```python
from build123d import *

# Parameters (mm, degrees)
SKETCH_W        = 90
SKETCH_H        = 130
PAD_DEPTH       = 3
PAD007_DEPTH    = 3
PAD006_DEPTH    = 3
SKETCH009_W     = 90
SKETCH009_H     = 130
PAD008_DEPTH    = 2
SKETCH010_R     = 19.0420352847
POCKET_DEPTH    = 10
CHAMFER_SIZE    = 1
SKETCH011_W     = 90
SKETCH011_H     = 4
POCKET001_DEPTH = 5


with BuildPart() as pad007:
    # Sketch → Pad (new body)
    with BuildSketch(Plane.XY):
        with Locations((45, 65)):
            Rectangle(SKETCH_W, SKETCH_H)
    extrude(amount=PAD_DEPTH)

    # Sketch006 → Pad007 (new body)
    with BuildSketch(Plane.XY.offset(3)):
        with BuildLine():
            Line((0, 0), (90, 0))
            Line((90, 0), (90, 31.200001))
            Line((90, 87.7297593266), (90, 31.200001))
            Line((63.384261619, 87.7297593266), (90, 87.7297593266))
            ThreePointArc((73.2419105019, 65.6401585516), (70.414665309, 77.6228043326), (63.384261619, 87.7297593266))
            ThreePointArc((61.470024, 41.9983394519), (70.1525128312, 52.4267750542), (73.2419105019, 65.6401585516))
            Line((61.470024, 31.2), (61.470024, 41.9983394519))
            Line((0, 31.2), (61.470024, 31.2))
            Line((0, 31.2), (0, 0))
        make_face()
    extrude(amount=PAD007_DEPTH)


with BuildPart() as pocket001:
    # Sketch008 → Pad006 (new body)
    with BuildSketch(Plane(origin=(90, 130, 3), x_dir=(-1, 0, 0), z_dir=(0, 0, 1))):
        with BuildLine():
            Line((0, 0), (90, 0))
            Line((90, 0), (90, 31.200001))
            Line((90, 87.7297593266), (90, 31.200001))
            Line((63.384261619, 87.7297593266), (90, 87.7297593266))
            ThreePointArc((73.2419105019, 65.6401585516), (70.414665309, 77.6228043326), (63.384261619, 87.7297593266))
            ThreePointArc((61.470024, 41.9983394519), (70.1525128312, 52.4267750542), (73.2419105019, 65.6401585516))
            Line((61.470024, 31.2), (61.470024, 41.9983394519))
            Line((0, 31.2), (61.470024, 31.2))
            Line((0, 31.2), (0, 0))
        make_face()
    extrude(amount=PAD006_DEPTH)

    # Fusion: union Pad007
    add(pad007.part)

    # Sketch009 → Pad008 (new body)
    with BuildSketch(Plane.XY.offset(6)):
        with Locations((45, 65)):
            Rectangle(SKETCH009_W, SKETCH009_H)
    extrude(amount=PAD008_DEPTH)

    # Sketch010 → Pocket (cut)
    with BuildSketch(Plane.XY.offset(8)):
        with Locations((45, 65)):
            Circle(SKETCH010_R)
    extrude(amount=-POCKET_DEPTH, mode=Mode.SUBTRACT)

    # Chamfer
    chamfer_edges = [pocket001.edges().sort_by_distance(p)[0] for p in [
        (25.957965, 65, 8),
    ]]
    chamfer(chamfer_edges, length=CHAMFER_SIZE)

    # Sketch011 → Pocket001 (cut)
    with BuildSketch(Plane.XZ):
        with Locations((45, 4.0113657125)):
            Rectangle(SKETCH011_W, SKETCH011_H)
    extrude(amount=-POCKET001_DEPTH, mode=Mode.SUBTRACT)


solid = pocket001.part
```
CAD build for the part. Positions are in the model's coordinates, mm. A direction names the side the tool comes from. Round coordinates to 2 decimals unless told otherwise and drop trailing zeros. Order: outer loops, then holes, each group sorted by start corner. A loop starts at its lowest first (then second) coordinate and runs counter-clockwise, first axis right, second up. Notation, with made-up numbers: (71.5, 8.5) -> (85.5, 8.5) arc R7 ccw to (85.5, 19.5) -> close; hole circle Ø1 at (-27, 88.5). An arc over 180 degrees is marked (long way). Write item = value, one per line.
(1) Drill centre lines: L1, parallel to Y at x = 45, z = 1.15; L2, parallel to Z at x = 25, y = 83; L3, parallel to X at y = 52.5, z = 0.75. Where is each one in solid material? Low to high.
Answers follow:
L1 = 0 to 45.96, 84.04 to 130
L2 = 0 to 3, 6 to 8
L3 = 0 to 30.64, 59.36 to 90
(2) 3-axis set-ups, long thin cutter, end or side, ignore diameter. For faces 1 (the flat face through (64.4, 65.5, 3)), 2 (the cylindrical face through (62.59, 57.71, 1.52)), 3 (the flat face through (44, 2, 2.011)), 4 (the flat face through (30, 31.2, 4)), 5 (the flat face through (77, 87.73, 4)): which of +Z, -Z, +X, -X, +Y, -Y reach the whole face in a straight line?
Answers follow:
face_1 = none
face_2 = +Z, -Z
face_3 = +X, -X, -Y
face_4 = -X
face_5 = +X
(3) Cut at A-A (x = 45). Write the cut outline in (y, z).
Answers follow:
outline = (0, 0) -> (45.96, 0) -> (45.96, 3) -> (31.2, 3) -> (31.2, 6) -> (45.96, 6) -> (45.96, 7) -> (44.96, 8) -> (0, 8) -> (0, 6.01) -> (5, 6.01) -> (5, 2.01) -> (0, 2.01) -> close; (84.04, 0) -> (130, 0) -> (130, 8) -> (85.04, 8) -> (84.04, 7) -> (84.04, 6) -> (98.8, 6) -> (98.8, 3) -> (84.04, 3) -> close
(4) Cut at B-B (x = 6.5). Write the cut outline in (y, z), plus the area to 3 significant figures.
Answers follow:
outline = (0, 0) -> (130, 0) -> (130, 8) -> (0, 8) -> (0, 6.01) -> (5, 6.01) -> (5, 2.01) -> (0, 2.01) -> close; hole (31.2, 3) -> (42.27, 3) -> (42.27, 6) -> (31.2, 6) -> close
area = 987 mm²
(5) Flat gauge pins, fed straight in: P1, Ø1.5, axis at y = 39.5, z = 4.5, coming from the -X side; P2, Ø1.5, axis at x = 19.5, z = 4.5, coming from the -Y side. Where does each tip first touch, or does it go through?
Answers follow:
P1 = 61.47
P2 = 5
(6) Pull direction X, two halves, no side cores. Call faces 6 (the flat face through (90, 64, 4)), 7 (the cylindrical face through (70.485, 77.464, 4.479)), 8 (the flat face through (44, 2, 6.011)): +X half, -X half, draft (parallel to the pull), parting line (faces both ways), or undercut.
Answers follow:
face_6 = +X half
face_7 = undercut
face_8 = draft
(7) Cut at D-D (x = 68). Write the cut outline in (y, z) (3 decimals).
Answers follow:
outline = (0, 0) -> (130, 0) -> (130, 8) -> (0, 8) -> (0, 6.011) -> (5, 6.011) -> (5, 2.011) -> (0, 2.011) -> close; hole (48.785, 3) -> (82.077, 3) -> (82.077, 6) -> (48.785, 6) -> close; hole (87.73, 3) -> (98.8, 3) -> (98.8, 6) -> (87.73, 6) -> close
(8) Cut at C-C (y = 91). Write the cut outline in (x, z), plus the area to 3 significant figures.
Answers follow:
outline = (0, 0) -> (90, 0) -> (90, 3) -> (28.53, 3) -> (28.53, 6) -> (90, 6) -> (90, 8) -> (0, 8) -> close
area = 536 mm²
